Build history of the part. All positions in model axes, mm. A direction names the side the tool comes from. Round coordinates to 2 decimals unless told otherwise and drop trailing zeros. Loops run counter-clockwise (first coordinate to the right, second up) from the corner with the lowest first, then second, coordinate; pieces in that order, holes last. Notation, with made-up numbers: M 55.25,87 L 64.25,87 A8 cw 64.25,99 Z; hole C -24,17.25 d4. An arc over 180 degrees is marked long. One line per item, written item: value.
Autodesk Inventor part; units mm, degrees
ref_plane "YZ Plane" through (0, 0, 0) normal (1, 0, 0) x (0, 1, 0)
ref_plane "XZ Plane" through (0, 0, 0) normal (0, 1, 0) x (-1, 0, 0)
ref_plane "XY Plane" through (0, 0, 0) normal (0, 0, 1) x (1, 0, 0)
sketch "Base Board" plane through (0, 0, 0) normal (0, 1, 0) x (-1, 0, 0)
  line L0 (5.0631, 4.2478) -> (-53.4369, 4.2478)
  line L1 (-53.4369, 4.2478) -> (-53.4369, -34.8522)
  line L2 (-53.4369, -34.8522) -> (5.0631, -34.8522)
  line L3 (5.0631, -34.8522) -> (5.0631, 4.2478)
  circle A0 centre (2.5631, 1.7478) radius 1.755
  circle A1 centre (-50.9369, 1.7478) radius 1.755
  point P0 (0, 0)
  dimension "d0" = 58.5
  dimension "d1" = 39.1
  dimension "d6" = 3.51
  dimension "d8" = 3.51
  dimension "d10" = 2.5
  dimension "d11" = 2.5
  dimension "d12" = 2.5
  dimension "d13" = 2.5
extrude "Base Extrusion" add sketch "Base Board" along normal blind 1.5
sketch "Sketch2" plane through (0, 1.5, 0) normal (0, 1, 0) x (1, 0, 0)
  line L0 (38.5869, -4.1507) -> (46.1869, -4.1507)
  line L1 (46.1869, -4.1507) -> (46.1869, 0.8493)
  line L2 (46.1869, 0.8493) -> (38.5869, 0.8493)
  line L3 (38.5869, 0.8493) -> (38.5869, -4.1507)
  line L4 (-5.0631, 34.8522) -> (-5.0631, -4.2478)
  line L5 (53.4369, -4.2478) -> (53.4369, 34.8522)
  dimension "d16" = 7.6
  dimension "d17" = 5
  dimension "d21" = 7.25
extrude "MicroUSB slot" add sketch "Sketch2" along normal blind 2.5
sketch "Sketch3" plane through (0, 1.5, 0) normal (0, 1, 0) x (1, 0, 0)
  line L0 (3.2869, -4.0967) -> (10.2869, -4.0967)
  line L1 (10.2869, -4.0967) -> (10.2869, -0.5967)
  line L2 (10.2869, -0.5967) -> (3.2869, -0.5967)
  line L3 (3.2869, -0.5967) -> (3.2869, -4.0967)
  line L4 (-5.0631, 34.8522) -> (-5.0631, -4.2478)
  point P0 (0, 0)
  dimension "d22" = 7
  dimension "d23" = 3.5
  dimension "d24" = 8.35
extrude "Reset Button" add sketch "Sketch3" along normal blind 3.35
sketch "Sketch4" plane through (0, 1.5, 0) normal (0, 1, 0) x (1, 0, 0)
  line L0 (43.4369, 31.6613) -> (18.4369, 31.6613)
  line L1 (18.4369, 31.6613) -> (18.4369, 34.6613)
  line L2 (18.4369, 34.6613) -> (43.4369, 34.6613)
  line L3 (43.4369, 34.6613) -> (43.4369, 31.6613)
  line L4 (53.4369, -4.2478) -> (53.4369, 34.8522)
  point P0 (0, 0)
  point P1 (43.4369, 33.1613)
  dimension "d27" = 25
  dimension "d28" = 3
  dimension "d29" = 10
extrude "Extrusion4" add sketch "Sketch4" along normal blind 8.55
properties part number "XDSEmulatorModule"
Item 1: Slice it at D-D, the plane y = 7.5. Give the cut face in (x, z), and give its area (3 significant figures).
Check values:
outline: M 18.44,-34.66 L 43.44,-34.66 L 43.44,-31.66 L 18.44,-31.66 Z
area: 75.0 mm2
Item 2: Pull direction Z, two halves, no side cores. Call faces 4 (the face through (-4.184, 0.74, 2.42)), 5 (the face through (7, 3, 0.597)), 6 (the face through (31, 10.05, -33)), 7 (the face through (52.69, 0.74, 1.67)): pulls with the +Z half, pulls with the -Z half, needs draft (parallel to the pull), parting line crosses it, or undercut.
Check values:
face 4: undercut
face 5: pulls with the -Z half
face 6: needs draft
face 7: undercut
Item 3: Wall check: line 1 along X through (y, z) = (1.75, 1.5); line 2 along Y through (x, z) = (50.5, -17); line 3 along X through (y, z) = (6, -32). Give the ranges that are in metal, low to high.
Check values:
line 1: x = 3.29 to 10.29, 38.59 to 46.19
line 2: y = 0 to 1.5
line 3: x = 18.44 to 43.44
Item 4: Which spindle directions (+Z, -Z, +X, -X, +Y, -Y) get a long thin tool onto all of the face, cutting with end or side? Do faces 1 (the face through (38.587, 3, 2)), 2 (the face through (7, 3, 4.097)), 3 (the face through (18.437, 6, -33)). Say none if no direction does.
Check values:
face 1: +Z, +Y
face 2: +Z, -X, +Y
face 3: +Z, -Z, -X, +Y
Item 5: Slice it at C-C, the plane z = -20.5. Give the cut face in (x, y), and give its area (4 significant figures).
Check values:
outline: M -5.06,0 L 53.44,0 L 53.44,1.5 L -5.06,1.5 Z
area: 87.75 mm2
Item 6: Slice it at A-A, the plane y = 2.25. Give the cut face in (x, z).
Check values:
outline: M 3.29,0.6 L 10.29,0.6 L 10.29,4.1 L 3.29,4.1 Z; M 18.44,-34.66 L 43.44,-34.66 L 43.44,-31.66 L 18.44,-31.66 Z; M 38.59,-0.85 L 46.19,-0.85 L 46.19,4.15 L 38.59,4.15 Z
Item 7: Slice it at B-B, the plane x = 42.5. Give the cut face in (y, z).
Check values:
outline: M 0,-34.85 L 1.5,-34.85 L 1.5,-34.66 L 10.05,-34.66 L 10.05,-31.66 L 1.5,-31.66 L 1.5,-0.85 L 4,-0.85 L 4,4.15 L 1.5,4.15 L 1.5,4.25 L 0,4.25 Z
Item 8: Drop flat-ended pins along their axis: P1, Ø6, axis at x = 19, y = 6, coming from the -Z side; P2, Ø3, axis at x = 6, z = 1.5, coming from the +Y side; P3, Ø1, axis at y = 3.5, z = 2, coming from the -X side. Give the stop position or say it passes through.
Check values:
P1: stops at z = -34.66
P2: stops at y = 4.85
P3: stops at x = 3.29
